Source: CAD feature listing. Evaluate the final solid. Frame: model axes, mm. Face numbers are marked on the shaded views. A direction names the side the tool comes from. Give positions to 0.01 mm unless a question says otherwise; leave off trailing zeros. Loops run counter-clockwise (first coordinate to the right, second up) from the corner with the lowest first, then second, coordinate; pieces in that order, holes last.
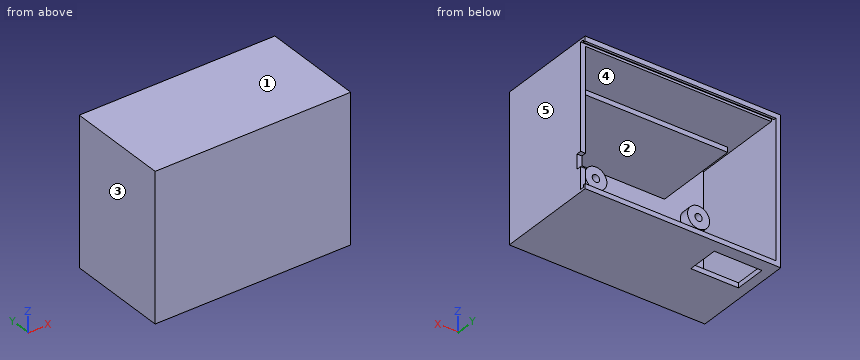
from build123d import *

# Parameters (mm, degrees)
SKIZZE1_W                       = 80
SKIZZE1_H                       = 60
AUFSATZ_LINEAR_AUSTRAGEN1_DEPTH = 42
WANDUNG1_T                      = -2
SKIZZE2_W                       = 60
SKIZZE2_H                       = 2
AUFSATZ_LINEAR_AUSTRAGEN2_DEPTH = 35
SKIZZE3_R                       = 4.5
SKIZZE3_R_2                     = 1.5
AUFSATZ_LINEAR_AUSTRAGEN3_DEPTH = 4
SKIZZE4_R                       = 4.5
SKIZZE4_R_2                     = 1.5
AUFSATZ_LINEAR_AUSTRAGEN4_DEPTH = 4
SCHNITT_LINEAR_AUSTRAGEN1_REACH = 82
SKIZZE6_W                       = 56
SKIZZE6_H                       = 2
SKIZZE7_W                       = 58
SKIZZE7_H                       = 1.5
SCHNITT_LINEAR_AUSTRAGEN2_DEPTH = 78
SCHNITT_LINEAR_AUSTRAGEN3_REACH = 82
SKIZZE8_W                       = 6
SKIZZE8_H                       = 2
SCHNITT_LINEAR_AUSTRAGEN5_REACH = 62
SKIZZE9_W                       = 19.5
SKIZZE9_H                       = 13


with BuildPart() as part:
    # Skizze1 → Aufsatz-Linear austragen1 (new body)
    with BuildSketch(Plane(origin=(0, 0, 0), x_dir=(1, 0, 0), z_dir=(0, 1, 0))):
        with Locations((40, 30)):
            Rectangle(SKIZZE1_W, SKIZZE1_H)
    extrude(amount=AUFSATZ_LINEAR_AUSTRAGEN1_DEPTH)

    # Wandung1
    wandung1_openings = [part.faces().sort_by_distance(p)[0] for p in [
        (40, 42, -30),
    ]]
    offset(amount=WANDUNG1_T, openings=wandung1_openings, kind=Kind.INTERSECTION)

    # Skizze2 → Aufsatz-Linear austragen2 (add)
    with BuildSketch(Plane(origin=(0, 2, 0), x_dir=(1, 0, 0), z_dir=(0, 1, 0))):
        with Locations((48, 18)):
            Rectangle(SKIZZE2_W, SKIZZE2_H)
    extrude(amount=AUFSATZ_LINEAR_AUSTRAGEN2_DEPTH)

    # Skizze3 → Aufsatz-Linear austragen3 (add)
    with BuildSketch(Plane(origin=(0, 2, 0), x_dir=(1, 0, 0), z_dir=(0, 1, 0))):
        with Locations((7, 24)):
            Circle(SKIZZE3_R)
        with Locations((7, 24)):
            Circle(SKIZZE3_R_2, mode=Mode.SUBTRACT)
        with Locations((23, 53)):
            Circle(SKIZZE3_R)
        with Locations((23, 53)):
            Circle(SKIZZE3_R_2, mode=Mode.SUBTRACT)
    extrude(amount=AUFSATZ_LINEAR_AUSTRAGEN3_DEPTH)

    # Skizze4 → Aufsatz-Linear austragen4 (add)
    with BuildSketch(Plane(origin=(0, 2, 0), x_dir=(1, 0, 0), z_dir=(0, 1, 0))):
        with Locations((49, 25)):
            Circle(SKIZZE4_R)
        with Locations((49, 25)):
            Circle(SKIZZE4_R_2, mode=Mode.SUBTRACT)
        with Locations((72, 48)):
            Circle(SKIZZE4_R)
        with Locations((72, 48)):
            Circle(SKIZZE4_R_2, mode=Mode.SUBTRACT)
    extrude(amount=AUFSATZ_LINEAR_AUSTRAGEN4_DEPTH)

    # Skizze6 → Schnitt-Linear austragen1 (cut, up to next)
    with BuildSketch(Plane(origin=(80, 0, 0), x_dir=(0, 0, -1), z_dir=(1, 0, 0)), mode=Mode.PRIVATE) as schnitt_linear_austragen1_sk1:
        with Locations((30, 41)):
            Rectangle(SKIZZE6_W, SKIZZE6_H)
    schnitt_linear_austragen1_tool1 = extrude(schnitt_linear_austragen1_sk1.sketch, amount=-SCHNITT_LINEAR_AUSTRAGEN1_REACH, mode=Mode.PRIVATE) & part.part
    add(schnitt_linear_austragen1_tool1.solids().sort_by_distance((80, 41, -30))[0], mode=Mode.SUBTRACT)

    # Skizze7 → Schnitt-Linear austragen2 (cut)
    with BuildSketch(Plane(origin=(80, 0, 0), x_dir=(0, 0, -1), z_dir=(1, 0, 0))):
        with Locations((30, 40.25)):
            Rectangle(SKIZZE7_W, SKIZZE7_H)
    extrude(amount=-SCHNITT_LINEAR_AUSTRAGEN2_DEPTH, mode=Mode.SUBTRACT)

    # Skizze8 → Schnitt-Linear austragen3 (cut, up to next)
    with BuildSketch(Plane(origin=(80, 0, 0), x_dir=(0, 0, -1), z_dir=(1, 0, 0)), mode=Mode.PRIVATE) as schnitt_linear_austragen3_sk1:
        with Locations((47, 38.5)):
            Rectangle(SKIZZE8_W, SKIZZE8_H)
    schnitt_linear_austragen3_tool1 = extrude(schnitt_linear_austragen3_sk1.sketch, amount=-SCHNITT_LINEAR_AUSTRAGEN3_REACH, mode=Mode.PRIVATE) & part.part
    add(schnitt_linear_austragen3_tool1.solids().sort_by_distance((80, 38.5, -47))[0], mode=Mode.SUBTRACT)

    # Skizze9 → Schnitt-Linear austragen5 (cut, up to next)
    with BuildSketch(Plane(origin=(0, 0, -60), x_dir=(-1, 0, 0), z_dir=(0, 0, -1)), mode=Mode.PRIVATE) as schnitt_linear_austragen5_sk1:
        with Locations((-13.75, 30.5)):
            Rectangle(SKIZZE9_W, SKIZZE9_H)
    schnitt_linear_austragen5_tool1 = extrude(schnitt_linear_austragen5_sk1.sketch, amount=-SCHNITT_LINEAR_AUSTRAGEN5_REACH, mode=Mode.PRIVATE) & part.part
    add(schnitt_linear_austragen5_tool1.solids().sort_by_distance((13.75, 30.5, -60))[0], mode=Mode.SUBTRACT)


solid = part.part
1) Reachability of the marked faces 4 and 5 from +Z, -Z, +X, -X, +Y, -Y: full face, straight path, thin tool, end or side. Return the list, or none.
Checks:
face 4: +Y
face 5: +Z, -Z, +X, +Y, -Y
2) Cut plane C-C (y = 19). Return loops of the section in (x, z).
Checks:
outline: (0, -60) - (80, -60) - (80, 0) - (0, 0) - close; hole (2, -58) - (78, -58) - (78, -19) - (18, -19) - (18, -17) - (78, -17) - (78, -2) - (2, -2) - close
3) Cut plane D-D (x = 63). Return loops of the section in (y, z).
Checks:
outline: (0, -60) - (42, -60) - (42, -58) - (41, -58) - (41, -59) - (39.5, -59) - (39.5, -58) - (2, -58) - (2, -19) - (37, -19) - (37, -17) - (2, -17) - (2, -2) - (39.5, -2) - (39.5, -1) - (41, -1) - (41, -2) - (42, -2) - (42, 0) - (0, 0) - close
4) Ray query, probe 1 along Z at (x, y) = (49, 4); probe 2 along Z at (x, y) = (27.5, 20.5); probe 3 along X at (y, z) = (5, -48). Return the intervals inside material, ascending.
Checks:
probe 1: z = -60 to -58, -29.5 to -26.5, -23.5 to -20.5, -19 to -17, -2 to 0
probe 2: z = -60 to -58, -19 to -17, -2 to 0
probe 3: x = 0 to 2, 67.5 to 70.5, 73.5 to 76.5, 78 to 80
5) Cut plane B-B (y = 34.5). Return loops of the section in (x, z).
Checks:
outline: (0, -60) - (4, -60) - (4, -58) - (2, -58) - (2, -2) - (78, -2) - (78, -17) - (18, -17) - (18, -19) - (78, -19) - (78, -58) - (23.5, -58) - (23.5, -60) - (80, -60) - (80, 0) - (0, 0) - close
6) Pull-direction query (Z, two-part tool) for the marked faces 1, 2 and 3; classes: released by +Z, released by -Z, zero draft, split by the parting line, or undercut.
Checks:
face 1: released by +Z
face 2: undercut
face 3: zero draft
7) Cut plane A-A (x = 7). Return loops of the section in (y, z).
Checks:
outline: (0, -60) - (24, -60) - (24, -58) - (2, -58) - (2, -28.5) - (6, -28.5) - (6, -25.5) - (2, -25.5) - (2, -22.5) - (6, -22.5) - (6, -19.5) - (2, -19.5) - (2, -2) - (39.5, -2) - (39.5, -1) - (41, -1) - (41, -2) - (42, -2) - (42, 0) - (0, 0) - close; (37, -60) - (42, -60) - (42, -58) - (41, -58) - (41, -59) - (39.5, -59) - (39.5, -58) - (37, -58) - close
8) Contact query for flat-ended pins moving along their axis: P1, Ø10, axis at x = 73.5, z = -50, coming from the +Y side; P2, Ø1, axis at y = 26, z = -18, coming from the -X side; P3, Ø6, axis at x = 60.5, z = -35, coming from the +Y side; P4, Ø2.5, axis at x = 23, z = -54, coming from the +Y side. Output: stop coordinate, or through.
Checks:
P1: stops at y = 39.5
P2: stops at x = 0
P3: stops at y = 2
P4: stops at y = 6
